Source: CAD feature listing. Evaluate the final solid. Frame: model axes, mm. Face numbers are marked on the shaded views. A direction names the side the tool comes from. Give positions to 0.01 mm unless a question says otherwise; leave off trailing zeros. Loops run counter-clockwise (first coordinate to the right, second up) from the corner with the lowest first, then second, coordinate; pieces in that order, holes last. Notation, with made-up numbers: M -27.75,79 L -12.75,79 A23 cw -12.75,113 Z; hole C 28.25,43 d8. An arc over 180 degrees is marked long. Answer in a Markdown table with one row per item.
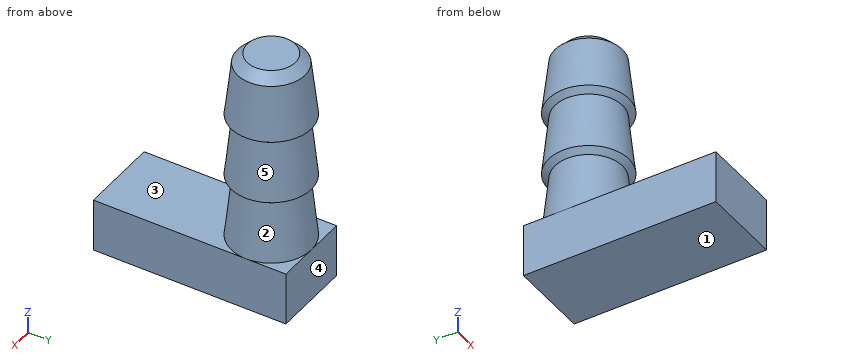
```python
from build123d import *

# Parameters (mm, degrees)
SKETCH002_W = 8.3
SKETCH002_H = 20
PAD_DEPTH   = 5.5


with BuildPart() as part:
    # Sketch002 → Pad (new body)
    with BuildSketch(Plane.XY):
        with Locations((0, -5.85)):
            Rectangle(SKETCH002_W, SKETCH002_H)
    extrude(amount=PAD_DEPTH)

    # Sketch003 → Revolution (revolve)
    with BuildSketch(Plane.YZ):
        Polygon((0, 5.5), (4.15, 5.5), (3.5, 11.666667), (4.15, 12.166667), (3.5, 18.333334), (4.15, 18.833334), (3.5, 24.500001), (2.5, 25.500001), (0, 25.500001), align=None)
    revolve(axis=Axis((0, 0, 0), (0, 0, 1)))


solid = part.part
```
1) Section B-B, the plane z = 21. Return loops of the section in (x, y), then the cut area to 3 significant figures.
Reply:
| item | result |
|---|---|
| outline | C 0,0 d7.8 |
| area | 47.8 mm² |
2) Material intervals for L1, parallel to Z at x = -2, y = -8; L2, parallel to X at y = 3, z = 8.25; L3, parallel to Z at x = 2, y = 2.25, sorted ascending.
Reply:
| item | result |
|---|---|
| L1 | z = 0 to 5.5 |
| L2 | x = -2.43 to 2.43 |
| L3 | z = 0 to 24.99 |
3) Pull-direction query (Z, two-part tool) for the marked faces 3, 4 and 5; classes: released by +Z, released by -Z, zero draft, split by the parting line, or undercut.
Reply:
| item | result |
|---|---|
| face 3 | released by +Z |
| face 4 | zero draft |
| face 5 | undercut |
4) Section A-A, the plane y = -5.25. Return loops of the section in (x, z), then the cut area to 4 significant figures.
Reply:
| item | result |
|---|---|
| outline | M -4.15,0 L 4.15,0 L 4.15,5.5 L -4.15,5.5 Z |
| area | 45.65 mm² |
5) Pin query (flat end, axial travel): pin 1 Ø2.5 at (x, y) = (0.5, -9) entering from +Z; pin 2 Ø2 at (y, z) = (-4, 20.5) entering from -X. Return the tip coordinate at first contact, or that it passes through.
Reply:
| item | result |
|---|---|
| pin 1 | stops at z = 5.5 |
| pin 2 | stops at x = -2.6 |
6) Section C-C, the plane z = 13.5. Return loops of the section in (x, y).
Reply:
| item | result |
|---|---|
| outline | C 0,0 d8.02 |
7) Set-up query: the marked faces 1 and 2. Return all of +Z, -Z, +X, -X, +Y, -Y with unobstructed straight access to the full face (end or side cutting, diameter ignored); none if empty.
Reply:
| item | result |
|---|---|
| face 1 | -Z, +X, -X, +Y, -Y |
| face 2 | none |
